Autodesk Inventor part; units mm, degrees
ref_plane "Work Plane1" through (0, 0, 10) normal (0, 0, 1) x (1, 0, 0)
ref_plane "YZ Plane" through (0, 0, 0) normal (1, 0, 0) x (0, 1, 0)
ref_plane "XZ Plane" through (0, 0, 0) normal (0, 1, 0) x (-1, 0, 0)
sketch "Sketch1" plane through (0, 0, 0) normal (0, 0, 1) x (1, 0, 0)
  line L0 (0, 0) -> (-30, 0)
  line L1 (-30, 0) -> (-30, -60)
  line L2 (0, 0) -> (-30, 0)
  line L3 (-30, 0) -> (-30, 3)
  line L4 (-30, 3) -> (0, 3)
  line L5 (0, 3) -> (0, 0)
  line L6 (-30, -60) -> (-33, -60)
  line L7 (-33, -60) -> (-33, 0)
  line L8 (-33, 0) -> (-30, 0)
  line L9 (-30, 0) -> (-30, -60)
  line L10 (-30, 3) -> (-33, 3)
  line L11 (-33, 3) -> (-33, 0)
  line L12 (-33, 0) -> (-30, 0)
  line L13 (-30, 0) -> (-30, 3)
  dimension "d0" = 30
  dimension "d1" = 60
  dimension "d2" = 3
  dimension "d3" = 3
extrude "Extrusion1" add sketch "Sketch1" along normal blind 20
sketch "Sketch2" plane through (-30, -60, 0) normal (1, 0, 0) x (0, 0, -1)
  line L0 (0, 63) -> (0, 0)
  line L1 (-20, 63) -> (-20, 0)
  line L2 (0, 0) -> (-20, 0)
  line L3 (-20, 0) -> (-20, 60)
  line L4 (-20, 60) -> (0, 60)
  line L5 (0, 60) -> (0, 0)
  line L6 (-10, 0) -> (-10, 8)
  line L7 (-10, 60) -> (-10, 52)
  circle A0 centre (-10, 52) radius 2.15
  circle A1 centre (-10, 8) radius 2.15
  dimension "d6" = 8
  dimension "d7" = 8
  dimension "d8" = 4.3
  dimension "d9" = 4.3
extrude "Extrusion2" cut sketch "Sketch2" against normal through all contours A0 | A1
sketch "Sketch3" plane through (-33, 3, 0) normal (0, 1, 0) x (1, 0, 0)
  line L0 (33, -20) -> (0, -20)
  line L1 (3, 0) -> (3, -20)
  line L2 (33, -20) -> (3, -20)
  line L3 (3, -20) -> (3, 0)
  line L4 (3, 0) -> (33, 0)
  line L5 (33, 0) -> (33, -20)
  line L6 (33, -10) -> (25, -10)
  line L7 (3, -10) -> (11, -10)
  circle A0 centre (11, -10) radius 2.15
  circle A1 centre (25, -10) radius 2.15
  dimension "d12" = 8
  dimension "d13" = 8
  dimension "d14" = 4.3
  dimension "d15" = 4.3
extrude "Extrusion3" cut sketch "Sketch3" against normal through all contours A1 | A0
ref_plane "Work Plane1" through (0, 0, 10) normal (0, 0, 1) x (1, 0, 0)
properties part number "BedBeltMount1"
Model file for the job. Use its own axes, mm. A direction names the side the tool comes from. Round coordinates to 2 decimals unless told otherwise and drop trailing zeros. Order: outer loops, then holes, each group sorted by start corner. A loop starts at its lowest first (then second) coordinate and runs counter-clockwise, first axis right, second up.
(1) Band-saw the part on D-D (y = -43). List the corners of the cut face in (x, z).
(2) Pin check, flat tips, straight feed: pin 1 (8 mm diameter, centred on x = -22.5, y = -49, fed in from +Z); pin 2 (10 mm diameter, centred on x = -12.5, z = 7, fed in from -Y); pin 3 (10 mm diameter, centred on y = -34, z = 10, fed in from +X). Stop position of each tip, or through.
(3) 3-axis set-ups, long thin cutter, end or side, ignore diameter. For faces 1 (the face through (-15, 0, 10)), 2 (the face through (-22.28, 1.52, 7.87)): which of +Z, -Z, +X, -X, +Y, -Y reach the whole face in a straight line?
(4) Drill centre lines: line 1 (X direction, y = 2.1, z = 10); line 2 (Y direction, x = -31.15, z = 10); line 3 (Z direction, x = -30.95, y = -52). Where is each one in solid material? Low to high.
(5) Pull direction Z, two halves, no side cores. Call faces 3 (the face through (-30, -30, 10)), 4 (the face through (-31.48, -5.87, 10.28)), 5 (the face through (-31, -21, 0)), 6 (the face through (-31, -21, 20)): released by +Z, released by -Z, zero draft, split by the parting line, or undercut.
(6) Band-saw the part on C-C (x = -31). List the corners of the cut face in (y, z), then the cut area to 3 significant figures.
(7) Band-saw the part on A-A (x = -8). List the corners of the cut face in (y, z), then the cut area to 3 significant figures.
(8) Band-saw the part on B-B (y = -8). List the corners of the cut face in (x, z), then the cut area to 3 significant figures.
Verdict:
1. outline: (-33, 0) - (-30, 0) - (-30, 20) - (-33, 20) - close
2. pin 1: passes through
2. pin 2: stops at y = 0
2. pin 3: stops at x = -30
3. face 1: +Z, -Z, +X, -Y
3. face 2: +Y, -Y
4. line 1: x = -33 to -24.15, -19.85 to -10.15, -5.85 to 0
4. line 2: y = -60 to -54.15, -49.85 to -10.15, -5.85 to 3
4. line 3: z = 0 to 7.85, 12.15 to 20
5. face 3: zero draft
5. face 4: undercut
5. face 5: released by -Z
5. face 6: released by +Z
6. outline: (-60, 0) - (3, 0) - (3, 20) - (-60, 20) - close; hole circle Ø4.3 at (-52, 10); hole circle Ø4.3 at (-8, 10)
6. area: 1,230 mm2
7. outline: (0, 0) - (3, 0) - (3, 7.85) - (0, 7.85) - close; (0, 12.15) - (3, 12.15) - (3, 20) - (0, 20) - close
7. area: 47.1 mm2
8. outline: (-33, 0) - (-30, 0) - (-30, 7.85) - (-33, 7.85) - close; (-33, 12.15) - (-30, 12.15) - (-30, 20) - (-33, 20) - close
8. area: 47.1 mm2
